from build123d import *

# Parameters (mm, degrees)
EXTRUDE_4_DEPTH     = 4
SKETCH_5_R          = 0.5
CUT_EXTRUDE_2_DEPTH = 4


with BuildPart() as part:
    # 草图1 → 凸台-拉伸4 (new body)
    with BuildSketch(Plane.XY):
        with BuildLine():
            Line((2, 3.464101615), (2, 2.236067977))
            ThreePointArc((2, 2.236067977), (2.738612788, 1.224744871), (3, 0))
            ThreePointArc((3, 0), (-1.224744871, -2.738612788), (-2, 2.236067977))
            Line((-2, 2.236067977), (-2, 3.464101615))
            ThreePointArc((-2, 3.464101615), (-2, -3.464101615), (4, 0))
            ThreePointArc((4, 0), (3.464101615, 2), (2, 3.464101615))
        make_face()
        with BuildLine():
            Line((1, 3), (0, 3))
            ThreePointArc((0, 3), (1.070466269, 2.802517077), (2, 2.236067977))
            Line((2, 2.236067977), (2, 3.464101615))
            ThreePointArc((2, 3.464101615), (1.513867916, 3.702459174), (1, 3.872983346))
            Line((1, 3.872983346), (1, 3))
        make_face()
        with BuildLine():
            ThreePointArc((-2, 2.236067977), (-1.070466269, 2.802517077), (0, 3))
            Line((0, 3), (-1, 3))
            Line((-1, 3), (-1, 3.872983346))
            ThreePointArc((-1, 3.872983346), (-1.513867916, 3.702459174), (-2, 3.464101615))
            Line((-2, 3.464101615), (-2, 2.236067977))
        make_face()
        with BuildLine():
            Line((-1, 3), (0, 3))
            Line((0, 3), (0, 4))
            ThreePointArc((0, 4), (-0.50401717, 3.968118785), (-1, 3.872983346))
            Line((-1, 3.872983346), (-1, 3))
        make_face()
        with BuildLine():
            Line((0, 4), (0, 3))
            Line((0, 3), (1, 3))
            Line((1, 3), (1, 3.872983346))
            ThreePointArc((1, 3.872983346), (0.50401717, 3.968118785), (0, 4))
        make_face()
        with BuildLine():
            Line((1, 8), (1, 3.872983346))
            ThreePointArc((1, 3.872983346), (1.513867916, 3.702459174), (2, 3.464101615))
            Line((2, 3.464101615), (2, 8))
            Line((2, 8), (1, 8))
        make_face()
        with BuildLine():
            ThreePointArc((-2, 3.464101615), (-1.513867916, 3.702459174), (-1, 3.872983346))
            Line((-1, 3.872983346), (-1, 8))
            Line((-1, 8), (-2, 8))
            Line((-2, 8), (-2, 3.464101615))
        make_face()
    extrude(amount=EXTRUDE_4_DEPTH)

    # 草图5 → 切除-拉伸2 (cut)
    with BuildSketch(Plane.ZY.offset(2)):
        with Locations((2, 6.5)):
            Circle(SKETCH_5_R)
    extrude(amount=-CUT_EXTRUDE_2_DEPTH, mode=Mode.SUBTRACT)


solid = part.part
Here's how the part is built. I have some questions about the finished solid (model axes, mm). A direction names the side the tool comes from. Give positions to 0.01 mm unless a question says otherwise; leave off trailing zeros. Loops run counter-clockwise (first coordinate to the right, second up) from the corner with the lowest first, then second, coordinate; pieces in that order, holes last. Notation, with made-up numbers: (21.5, 82.5) -> (29.5, 82.5) arc R13 cw to (29.5, 99.5) -> close; hole circle Ø6 at (21, 7). An arc over 180 degrees is marked (long way). Answer as a JSON object with one key per item and string values. Group by question number.
Item 1: Imagine slicing it at C-C on y = 6.5. Write out the boundary of the cut face in (x, z).
Item 2: Thinking about a two-plate mould opening in Z: for faces 5 (the cylindrical face through (-1.507, 6.012, 1.892)), 6 (the flat face through (1, 3, 4)), 7 (the flat face through (-1, 5, 2)), which applies, pulls with the +Z half, pulls with the -Z half, needs draft (parallel to the pull), parting line crosses it, or undercut?
Item 3: On a 3-axis mill with a long thin cutter (end or side, diameter ignored), from which of +Z, -Z, +X, -X, +Y, -Y can I reach the whole of each face in a straight line? I mean faces 1 (the flat face through (2, 5.7, 2)), 2 (the flat face through (1, 5.5, 2)), 3 (the flat face through (1.5, 8, 2)), 4 (the flat face through (-2, 5.8, 2)). Say none if no direction works.
Item 4: Imagine slicing it at A-A on z = 2. Write out the boundary of the cut face in (x, y), then the cut area to 3 significant figures.
Item 5: Will these pins go through, and if not, where does the flat tip stop? pin 1 (1.2 mm diameter, centred on y = 6, z = 3, fed in from +X); pin 2 (1.5 mm diameter, centred on x = 1, z = 2, fed in from -Y); pin 3 (1.2 mm diameter, centred on y = 5, z = 2, fed in from -X).
Item 6: Imagine slicing it at D-D on y = 4.75. Write out the boundary of the cut face in (x, z), then the cut area to 3 significant figures.
Item 7: Imagine slicing it at B-B on x = 2.25. Write out the boundary of the cut face in (y, z).
Item 8: I need wall thicknesses on L1, parallel to X at y = 5.25, z = 1.6; L2, parallel to Y at x = 1.5, z = 2; L3, parallel to Y at x = -0.5, z = 2.65. Which ranges of each line are inside material? Lowest first, please.
Answer list:
{
 "1": {"outline": "(-2, 0) -> (-1, 0) -> (-1, 1.5) -> (-2, 1.5) -> close; (-2, 2.5) -> (-1, 2.5) -> (-1, 4) -> (-2, 4) -> close; (1, 0) -> (2, 0) -> (2, 1.5) -> (1, 1.5) -> close; (1, 2.5) -> (2, 2.5) -> (2, 4) -> (1, 4) -> close"},
 "2": {"face 5": "undercut", "face 6": "pulls with the +Z half", "face 7": "needs draft"},
 "3": {"face 1": "+Z, -Z, +X, +Y", "face 2": "+Z, -Z, +Y", "face 3": "+Z, -Z, +X, -X, +Y", "face 4": "+Z, -Z, -X, +Y"},
 "4": {"outline": "(-2, 3.46) arc R4 ccw (long way) to (2, 3.46) -> (2, 6) -> (1, 6) -> (1, 3.87) arc R4 ccw to (-1, 3.87) -> (-1, 6) -> (-2, 6) -> close; (-2, 7) -> (-1, 7) -> (-1, 8) -> (-2, 8) -> close; (1, 7) -> (2, 7) -> (2, 8) -> (1, 8) -> close; hole circle Ø6 at (0, 0)", "area": "28.6 mm2"},
 "5": {"pin 1": "stops at x = 2", "pin 2": "stops at y = -3.99", "pin 3": "stops at x = -2"},
 "6": {"outline": "(-2, 0) -> (-1, 0) -> (-1, 4) -> (-2, 4) -> close; (1, 0) -> (2, 0) -> (2, 4) -> (1, 4) -> close", "area": "8.00 mm2"},
 "7": {"outline": "(-3.31, 0) -> (-1.98, 0) -> (-1.98, 4) -> (-3.31, 4) -> close; (1.98, 0) -> (3.31, 0) -> (3.31, 4) -> (1.98, 4) -> close"},
 "8": {"L1": "x = -2 to -1, 1 to 2", "L2": "y = -3.71 to -2.6, 2.6 to 6, 7 to 8", "L3": "y = -3.97 to -2.96, 2.96 to 3.97"}
}
